Drawing for the job (mm, zero at the part's lowest x, y, z). Coordinates: 2 decimals unless noted, no trailing zeros. Write each loop counter-clockwise with the first axis right and the second up, starting at its lowest first coordinate (ties: lowest second). Pieces come first, ordered by that corner, then holes. Notation, with made-up numbers: (17, 5) -> (35, 5) arc R30 cw to (35, 31) -> close; hole circle Ø10 at (55, 83). An arc over 180 degrees is marked (long way). Write item = value, one per line. Start each with the question number.
Q1. Pin check, flat tips, straight feed: P1, Ø1.2, axis at y = 1.5, z = 1.5, coming from the -X side; P2, Ø2, axis at x = 41.5, z = 0.5, coming from the -Y side. Stop position of each tip, or through.
Q2. Probe line 1 (X direction, y = 1.4, z = 3.6); line 2 (X direction, y = 0.6, z = 0.9); line 3 (Y direction, x = 41, z = 1.85). List the from-to ranges inside material, lowest first.
Q3. Band-saw the part on A-A, the plane x = 39. List the corners of the cut face in (y, z).
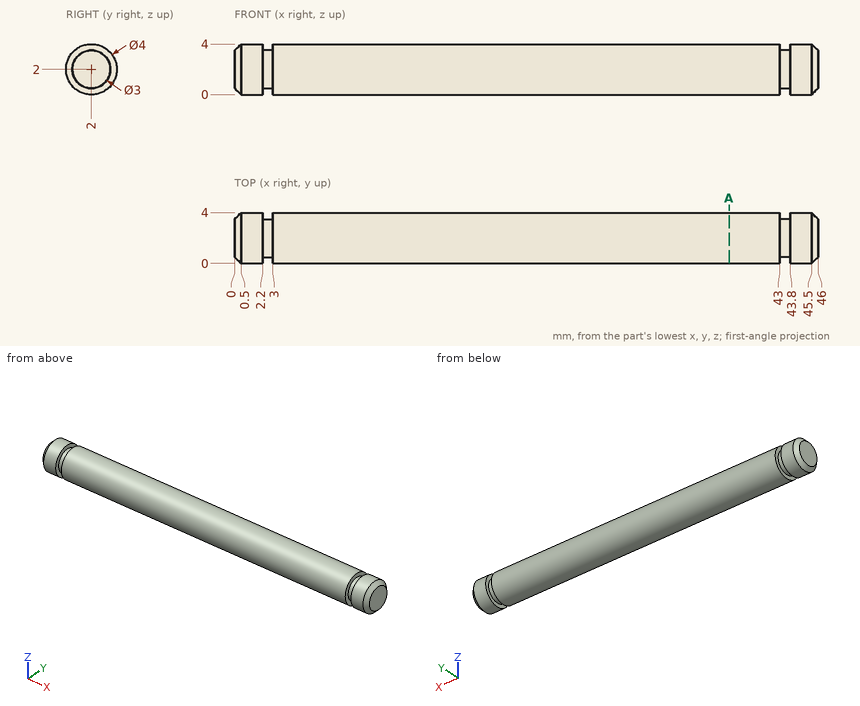
Ans:
q1.P1 = 0
q1.P2 = 0.06
q2.line_1 = 0.21 to 2.2, 3 to 43, 43.8 to 45.79
q2.line_2 = 0.28 to 2.2, 3 to 43, 43.8 to 45.72
q2.line_3 = 0.01 to 3.99
q3.outline = circle Ø4 at (2, 2)
